```python
from build123d import *

# Parameters (mm, degrees)
SKETCH1_W           = 106
SKETCH1_H           = 10
BOSS_EXTRUDE1_DEPTH = 7
FILLET1_R           = 5
SKETCH2_R           = 1.5
CUT_EXTRUDE1_DEPTH  = 54.693575035
SKETCH3_R           = 1.5
BOSS_EXTRUDE2_DEPTH = 3
FILLET2_R           = 5
FILLET3_R           = 5
FILLET4_R           = 5
SKETCH4_W           = 33.5
SKETCH4_H           = 10
BOSS_EXTRUDE3_DEPTH = 1


with BuildPart() as part:
    # Sketch1 → Boss-Extrude1 (new body)
    with BuildSketch(Plane.XY):
        Rectangle(SKETCH1_W, SKETCH1_H)
    extrude(amount=BOSS_EXTRUDE1_DEPTH)

    # Fillet1
    fillet1_edges = [part.edges().sort_by_distance(p)[0] for p in [
        (-53, -5, 3.5),
        (53, -5, 3.5),
        (53, 5, 3.5),
        (-53, 5, 3.5),
    ]]
    fillet(fillet1_edges, radius=FILLET1_R - 0.0001)  # a hair under: the kernel refuses the full size

    # Sketch2 → Cut-Extrude1 (cut, through all)
    with BuildSketch(Plane.XY.offset(7)):
        with Locations((-48, 0)):
            Circle(SKETCH2_R)
        with Locations((48, 0)):
            Circle(SKETCH2_R)
        Circle(SKETCH2_R)
    extrude(amount=-CUT_EXTRUDE1_DEPTH, mode=Mode.SUBTRACT)

    # Sketch3 → Boss-Extrude2 (add)
    # profile 1 of 2: a face of its own
    with BuildSketch(Plane.XY.offset(7)):
        with BuildLine():
            Line((7, 11), (7, 5))
            Line((7, 5), (13, 5))
            Line((13, 5), (13, 11))
            ThreePointArc((13, 11), (10, 14), (7, 11))
        make_face()
        with Locations((10, 11)):
            Circle(SKETCH3_R, mode=Mode.SUBTRACT)
    # profile 2 of 2: a face of its own
    with BuildSketch(Plane.XY.offset(7)):
        with BuildLine():
            Line((-7, 11), (-7, 5))
            Line((-7, 5), (-13, 5))
            Line((-13, 5), (-13, 11))
            ThreePointArc((-13, 11), (-10, 14), (-7, 11))
        make_face()
        with Locations((-10, 11)):
            Circle(SKETCH3_R, mode=Mode.SUBTRACT)
    extrude(amount=-BOSS_EXTRUDE2_DEPTH)

    # Fillet2
    fillet2_edges = [part.edges().sort_by_distance(p)[0] for p in [
        (-13, 5, 5.5),
    ]]
    fillet(fillet2_edges, radius=FILLET2_R)

    # Fillet3
    fillet3_edges = [part.edges().sort_by_distance(p)[0] for p in [
        (7, 5, 5.5),
        (-7, 5, 5.5),
    ]]
    fillet(fillet3_edges, radius=FILLET3_R)

    # Fillet4
    fillet4_edges = [part.edges().sort_by_distance(p)[0] for p in [
        (13, 5, 5.5),
    ]]
    fillet(fillet4_edges, radius=FILLET4_R)

    # Sketch4 → Boss-Extrude3 (add)
    with BuildSketch(Plane(origin=(0, 0, 0), x_dir=(-1, 0, 0), z_dir=(0, 0, -1))):
        with Locations((-24, 0)):
            Rectangle(SKETCH4_W, SKETCH4_H)
        with Locations((24, 0)):
            Rectangle(SKETCH4_W, SKETCH4_H)
    extrude(amount=BOSS_EXTRUDE3_DEPTH)


solid = part.part
```
CAD build for the part. Positions are in the model's coordinates, mm. A direction names the side the tool comes from. Round coordinates to 2 decimals unless told otherwise and drop trailing zeros. Loops run counter-clockwise (first coordinate to the right, second up) from the corner with the lowest first, then second, coordinate; pieces in that order, holes last. Notation, with made-up numbers: (20, 50) - (61, 50) arc R5 ccw to (61, 57) - close; hole circle Ø10 at (81, 13). An arc over 180 degrees is marked (long way). Return JSON: item names as keys, results as strings. Group by question number.
Q1. Tool access for faces 1 (the face through (45, 0, 0)), 2 (the face through (-1, 5, 3)), 3 (the face through (-10, 9, 4)): list every direction of +Z, -Z, +X, -X, +Y, -Y with a clear straight run to the whole face (end or side of a thin tool).
Q2. Band-saw the part on B-B on z = 6. Give the number of separate pieces and of enclosed holes in the cut face, plus the area to 3 significant figures.
Q3. Band-saw the part on D-D on x = 42. Give the cut face in (y, z).
Q4. Two-plate mould, pull along Y, no slides. Class faces 4 (the face through (2, 0, 0)), 5 (the face through (46.5, 0.07, 3.55)), 6 (the face through (6, 7, 5)), 7 (the face through (8.5, 11.07, 5.52)): +Y half, -Y half, draft (parallel to the pull), parting line (faces both ways), or undercut.
Q5. Band-saw the part on A-A on x = -10. Give the cut face in (y, z).
Q6. Flat gauge pins, fed straight in: pin 1 Ø0.5 at (y, z) = (-1, -0.5) entering from +X; pin 2 Ø2.5 at (x, y) = (-13.5, 9.5) entering from -Z; pin 3 Ø0.8 at (y, z) = (-0.5, -0.5) entering from -X. Where does each tip first touch, or does it go through?
Q7. Drill centre lines: line 1 along Y through (x, z) = (48, 2.75); line 2 along X through (y, z) = (-1.25, 4.5); line 3 along X through (y, z) = (0.75, 2.75). Where is each one in solid material? Low to high. Write a range as [from, to].
Q8. Band-saw the part on C-C on y = 7.5. Give the cut face in (x, z), plus the area to 3 significant figures.
Solutions:
{
 "1": {"face 1": "-Z, +X, +Y, -Y", "face 2": "-Z, +Y", "face 3": "-Z, +X, -X, +Y"},
 "2": {"separate pieces": "1", "enclosed holes": "5", "area": "1,120 mm^2"},
 "3": {"outline": "(-5, 0) - (5, 0) - (5, 7) - (-5, 7) - close"},
 "4": {"face 4": "draft", "face 5": "undercut", "face 6": "+Y half", "face 7": "undercut"},
 "5": {"outline": "(-5, -1) - (5, -1) - (5, 4) - (9.5, 4) - (9.5, 7) - (-5, 7) - close; (12.5, 4) - (14, 4) - (14, 7) - (12.5, 7) - close"},
 "6": {"pin 1": "stops at x = 40.75", "pin 2": "stops at z = 4", "pin 3": "stops at x = -40.75"},
 "7": {"line 1": "y = [-5, -1.5], [1.5, 5]", "line 2": "x = [-52.84, -48.83], [-47.17, -0.83], [0.83, 47.17], [48.83, 52.84]", "line 3": "x = [-52.94, -49.3], [-46.7, -1.3], [1.3, 46.7], [49.3, 52.94]"},
 "8": {"outline": "(-13.67, 4) - (-6.33, 4) - (-6.33, 7) - (-13.67, 7) - close; (6.33, 4) - (13.67, 4) - (13.67, 7) - (6.33, 7) - close", "area": "44.0 mm^2"}
}
